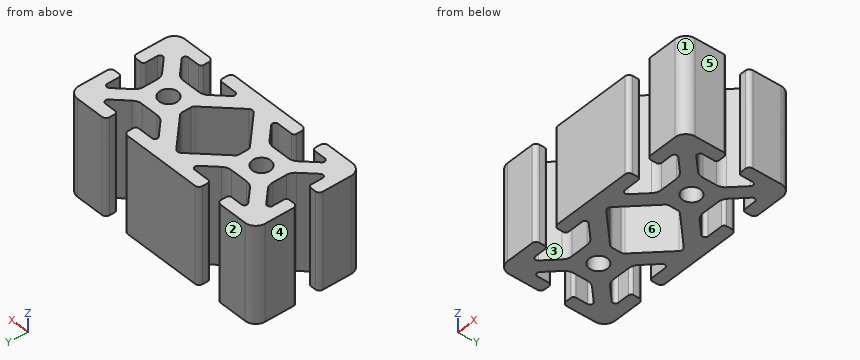
from build123d import *

# Parameters (mm, degrees)
SKETCH1_R           = 3.4
BOSS_EXTRUDE1_DEPTH = 36


with BuildPart() as part:
    # Sketch1 → Boss-Extrude1 (new body)
    with BuildSketch(Plane.XY):
        with BuildLine():
            Line((-36, -20), (-25.5, -20))
            ThreePointArc((-25.5, -20), (-24.439339828, -19.560660172), (-24, -18.5))
            Line((-24, -18.5), (-24, -16.5))
            ThreePointArc((-24, -16.5), (-24.292893219, -15.792893219), (-25, -15.5))
            Line((-25, -15.5), (-29.307617972, -15.5))
            ThreePointArc((-29.307617972, -15.5), (-30.305407867, -14.833298107), (-30.071293296, -13.656324676))
            Line((-30.071293296, -13.656324676), (-25.336541495, -8.921572875))
            ThreePointArc((-25.336541495, -8.921572875), (-24.038848099, -8.05448187), (-22.50811437, -7.75))
            Line((-22.50811437, -7.75), (-15.987648609, -7.75))
            ThreePointArc((-15.987648609, -7.75), (-14.45691488, -8.05448187), (-13.159221485, -8.921572875))
            Line((-13.159221485, -8.921572875), (-8.424469683, -13.656324676))
            ThreePointArc((-8.424469683, -13.656324676), (-8.190355112, -14.833298107), (-9.188145007, -15.5))
            Line((-9.188145007, -15.5), (-15, -15.5))
            ThreePointArc((-15, -15.5), (-15.707106781, -15.792893219), (-16, -16.5))
            Line((-16, -16.5), (-16, -18.5))
            ThreePointArc((-16, -18.5), (-15.560660172, -19.560660172), (-14.5, -20))
            Line((-14.5, -20), (14.5, -20))
            ThreePointArc((14.5, -20), (15.560660172, -19.560660172), (16, -18.5))
            Line((16, -18.5), (16, -16.5))
            ThreePointArc((16, -16.5), (15.707106781, -15.792893219), (15, -15.5))
            Line((15, -15.5), (9.188145007, -15.5))
            ThreePointArc((9.188145007, -15.5), (8.190355112, -14.833298107), (8.424469683, -13.656324676))
            Line((8.424469683, -13.656324676), (13.159221485, -8.921572875))
            ThreePointArc((13.159221485, -8.921572875), (14.45691488, -8.05448187), (15.987648609, -7.75))
            Line((15.987648609, -7.75), (22.50811437, -7.75))
            ThreePointArc((22.50811437, -7.75), (24.038848099, -8.05448187), (25.336541495, -8.921572875))
            Line((25.336541495, -8.921572875), (30.071293296, -13.656324676))
            ThreePointArc((30.071293296, -13.656324676), (30.305407867, -14.833298107), (29.307617972, -15.5))
            Line((29.307617972, -15.5), (25, -15.5))
            ThreePointArc((25, -15.5), (24.292893219, -15.792893219), (24, -16.5))
            Line((24, -16.5), (24, -18.5))
            ThreePointArc((24, -18.5), (24.439339828, -19.560660172), (25.5, -20))
            Line((25.5, -20), (36, -20))
            ThreePointArc((36, -20), (38.828427125, -18.828427125), (40, -16))
            Line((40, -16), (40, -5.5))
            ThreePointArc((40, -5.5), (39.560660172, -4.439339828), (38.5, -4))
            Line((38.5, -4), (36.5, -4))
            ThreePointArc((36.5, -4), (35.792893219, -4.292893219), (35.5, -5))
            Line((35.5, -5), (35.5, -9.307617972))
            ThreePointArc((35.5, -9.307617972), (34.833298107, -10.305407867), (33.656324676, -10.071293296))
            Line((33.656324676, -10.071293296), (28.921572875, -5.336541495))
            ThreePointArc((28.921572875, -5.336541495), (28.05448187, -4.038848099), (27.75, -2.50811437))
            Line((27.75, -2.50811437), (27.75, 2.50811437))
            ThreePointArc((27.75, 2.50811437), (28.05448187, 4.038848099), (28.921572875, 5.336541495))
            Line((28.921572875, 5.336541495), (33.656324676, 10.071293296))
            ThreePointArc((33.656324676, 10.071293296), (34.833298107, 10.305407867), (35.5, 9.307617972))
            Line((35.5, 9.307617972), (35.5, 5))
            ThreePointArc((35.5, 5), (35.792893219, 4.292893219), (36.5, 4))
            Line((36.5, 4), (38.5, 4))
            ThreePointArc((38.5, 4), (39.560660172, 4.439339828), (40, 5.5))
            Line((40, 5.5), (40, 16))
            ThreePointArc((40, 16), (38.828427125, 18.828427125), (36, 20))
            Line((36, 20), (25.5, 20))
            ThreePointArc((25.5, 20), (24.439339828, 19.560660172), (24, 18.5))
            Line((24, 18.5), (24, 16.5))
            ThreePointArc((24, 16.5), (24.292893219, 15.792893219), (25, 15.5))
            Line((25, 15.5), (29.307617972, 15.5))
            ThreePointArc((29.307617972, 15.5), (30.305407867, 14.833298107), (30.071293296, 13.656324676))
            Line((30.071293296, 13.656324676), (25.336541495, 8.921572875))
            ThreePointArc((25.336541495, 8.921572875), (24.038848099, 8.05448187), (22.50811437, 7.75))
            Line((22.50811437, 7.75), (15.987648609, 7.75))
            ThreePointArc((15.987648609, 7.75), (14.45691488, 8.05448187), (13.159221485, 8.921572875))
            Line((13.159221485, 8.921572875), (8.424469683, 13.656324676))
            ThreePointArc((8.424469683, 13.656324676), (8.190355112, 14.833298107), (9.188145007, 15.5))
            Line((9.188145007, 15.5), (15, 15.5))
            ThreePointArc((15, 15.5), (15.707106781, 15.792893219), (16, 16.5))
            Line((16, 16.5), (16, 18.5))
            ThreePointArc((16, 18.5), (15.560660172, 19.560660172), (14.5, 20))
            Line((14.5, 20), (-14.5, 20))
            ThreePointArc((-14.5, 20), (-15.560660172, 19.560660172), (-16, 18.5))
            Line((-16, 18.5), (-16, 16.5))
            ThreePointArc((-16, 16.5), (-15.707106781, 15.792893219), (-15, 15.5))
            Line((-15, 15.5), (-9.188145007, 15.5))
            ThreePointArc((-9.188145007, 15.5), (-8.190355112, 14.833298107), (-8.424469683, 13.656324676))
            Line((-8.424469683, 13.656324676), (-13.159221485, 8.921572875))
            ThreePointArc((-13.159221485, 8.921572875), (-14.45691488, 8.05448187), (-15.987648609, 7.75))
            Line((-15.987648609, 7.75), (-22.50811437, 7.75))
            ThreePointArc((-22.50811437, 7.75), (-24.038848099, 8.05448187), (-25.336541495, 8.921572875))
            Line((-25.336541495, 8.921572875), (-30.071293296, 13.656324676))
            ThreePointArc((-30.071293296, 13.656324676), (-30.305407867, 14.833298107), (-29.307617972, 15.5))
            Line((-29.307617972, 15.5), (-25, 15.5))
            ThreePointArc((-25, 15.5), (-24.292893219, 15.792893219), (-24, 16.5))
            Line((-24, 16.5), (-24, 18.5))
            ThreePointArc((-24, 18.5), (-24.439339828, 19.560660172), (-25.5, 20))
            Line((-25.5, 20), (-36, 20))
            ThreePointArc((-36, 20), (-38.828427125, 18.828427125), (-40, 16))
            Line((-40, 16), (-40, 5.5))
            ThreePointArc((-40, 5.5), (-39.560660172, 4.439339828), (-38.5, 4))
            Line((-38.5, 4), (-36.5, 4))
            ThreePointArc((-36.5, 4), (-35.792893219, 4.292893219), (-35.5, 5))
            Line((-35.5, 5), (-35.5, 9.307617972))
            ThreePointArc((-35.5, 9.307617972), (-34.833298107, 10.305407867), (-33.656324676, 10.071293296))
            Line((-33.656324676, 10.071293296), (-28.921572875, 5.336541495))
            ThreePointArc((-28.921572875, 5.336541495), (-28.05448187, 4.038848099), (-27.75, 2.50811437))
            Line((-27.75, 2.50811437), (-27.75, -2.50811437))
            ThreePointArc((-27.75, -2.50811437), (-28.05448187, -4.038848099), (-28.921572875, -5.336541495))
            Line((-28.921572875, -5.336541495), (-33.656324676, -10.071293296))
            ThreePointArc((-33.656324676, -10.071293296), (-34.833298107, -10.305407867), (-35.5, -9.307617972))
            Line((-35.5, -9.307617972), (-35.5, -5))
            ThreePointArc((-35.5, -5), (-35.792893219, -4.292893219), (-36.5, -4))
            Line((-36.5, -4), (-38.5, -4))
            ThreePointArc((-38.5, -4), (-39.560660172, -4.439339828), (-40, -5.5))
            Line((-40, -5.5), (-40, -16))
            ThreePointArc((-40, -16), (-38.828427125, -18.828427125), (-36, -20))
        make_face()
        with Locations((-20, 0)):
            Circle(SKETCH1_R, mode=Mode.SUBTRACT)
        with Locations((20, 0)):
            Circle(SKETCH1_R, mode=Mode.SUBTRACT)
        with BuildLine():
            Line((-11.810660172, 2.760660172), (-1.060660172, 13.510660172))
            ThreePointArc((-1.060660172, 13.510660172), (0, 13.95), (1.060660172, 13.510660172))
            Line((1.060660172, 13.510660172), (11.810660172, 2.760660172))
            ThreePointArc((11.810660172, 2.760660172), (12.135819299, 2.274025149), (12.25, 1.7))
            Line((12.25, 1.7), (12.25, -1.7))
            ThreePointArc((12.25, -1.7), (12.135819299, -2.274025149), (11.810660172, -2.760660172))
            Line((11.810660172, -2.760660172), (1.060660172, -13.510660172))
            ThreePointArc((1.060660172, -13.510660172), (0, -13.95), (-1.060660172, -13.510660172))
            Line((-1.060660172, -13.510660172), (-11.810660172, -2.760660172))
            ThreePointArc((-11.810660172, -2.760660172), (-12.135819299, -2.274025149), (-12.25, -1.7))
            Line((-12.25, -1.7), (-12.25, 1.7))
            ThreePointArc((-12.25, 1.7), (-12.135819299, 2.274025149), (-11.810660172, 2.760660172))
        make_face(mode=Mode.SUBTRACT)
    extrude(amount=BOSS_EXTRUDE1_DEPTH)


solid = part.part
For this review, take the finished solid that the model builds, in its own axes (mm). Face numbers are marked on the shaded views. A direction names the side the tool comes from. Round coordinates to 2 decimals unless told otherwise and drop trailing zeros. Write each loop counter-clockwise with the first axis right and the second up, starting at its lowest first coordinate (ties: lowest second). Pieces come first, ordered by that corner, then holes. Notation, with made-up numbers: (57, 53.25) -> (65, 53.25) arc R7 ccw to (65, 64.25) -> close; hole circle Ø10 at (-8, -19.5). An arc over 180 degrees is marked (long way). Use CSV: the item, a comma, the result in double quotes.
(1) Clearance check with flat-ended pins moving along their axes: P1, Ø2, axis at x = 18.5, z = 16, coming from the -Y side; P2, Ø1, axis at y = -17.5, z = 12.5, coming from the +X side; P3, Ø2, axis at x = -37.5, z = 17.5, coming from the +Y side. State where each tip first meets the part, or that it passes through.
Computed values:
P1,"y = -7.75"
P2,"x = 39.87"
P3,"y = 19.97"
(2) Draft analysis for pull direction Y (two halves, no side actions). For the marked faces 1, 2, 3 and 4, state which applies: +Y half, -Y half, draft (parallel to the pull), parting line (faces both ways), or undercut.
Computed values:
face 1,"-Y half"
face 2,"+Y half"
face 3,"undercut"
face 4,"draft"
(3) Consider section A-A, the plane y = 0. Give the boundary of the cut face in (x, z).
Computed values:
outline,"(-27.75, 0) -> (-23.4, 0) -> (-23.4, 36) -> (-27.75, 36) -> close; (-16.6, 0) -> (-12.25, 0) -> (-12.25, 36) -> (-16.6, 36) -> close; (12.25, 0) -> (16.6, 0) -> (16.6, 36) -> (12.25, 36) -> close; (23.4, 0) -> (27.75, 0) -> (27.75, 36) -> (23.4, 36) -> close"
(4) Consider section D-D, the plane y = -12. Give the boundary of the cut face in (x, z).
Computed values:
outline,"(-40, 0) -> (-28.41, 0) -> (-28.41, 36) -> (-40, 36) -> close; (-10.08, 0) -> (-2.57, 0) -> (-2.57, 36) -> (-10.08, 36) -> close; (2.57, 0) -> (10.08, 0) -> (10.08, 36) -> (2.57, 36) -> close; (28.41, 0) -> (40, 0) -> (40, 36) -> (28.41, 36) -> close"
(5) Consider section B-B, the plane x = 20. Give the boundary of the cut face in (y, z), plus the area to 3 significant figures.
Computed values:
outline,"(-7.75, 0) -> (-3.4, 0) -> (-3.4, 36) -> (-7.75, 36) -> close; (3.4, 0) -> (7.75, 0) -> (7.75, 36) -> (3.4, 36) -> close"
area,"313 mm²"
(6) Consider section C-C, the plane z = 12. Give the number of separate pieces and of enclosed holes in the cut face, plus the area to 3 significant figures.
Computed values:
separate pieces,"1"
enclosed holes,"3"
area,"1,700 mm²"
(7) To check wall thickness, follow L1, parallel to X at y = 14.5, z = 26.5; L2, parallel to Y at x = -20, z = 20; L3, parallel to Y at x = 26, z = 3.5. State the ranges of each line that lie inside material, in increasing order. Write a range as [from, to].
Computed values:
L1,"[-40, -30.38], [-8.11, 8.11], [30.38, 40]"
L2,"[-7.75, -3.4], [3.4, 7.75]"
L3,"[-20, -15.5], [-9.59, 9.59], [15.5, 20]"
(8) For the marked faces 5 and 6, list the 3-axis set-ups (+Z, -Z, +X, -X, +Y, -Y) from which the entire face can be reached by the end or side of a thin tool; tool diameter is ignored.
Computed values:
face 5,"+Z, -Z, +X, +Y, -Y"
face 6,"+Z, -Z"
